The model under review builds one solid part; all positions refer to its coordinate system, in mm. A direction names the side the tool comes from. Give positions to 0.01 mm unless a question says otherwise; leave off trailing zeros. Order: outer loops, then holes, each group sorted by start corner. A loop starts at its lowest first (then second) coordinate and runs counter-clockwise, first axis right, second up. Notation, with made-up numbers: (-36, 3.25) - (-13, 3.25) arc R17 cw to (-13, 26.25) - close; hole circle Ø5 at (16, 65). An arc over 180 degrees is marked (long way). Use CSV: the item, a comma, the result in double quotes. Start each with the question number.
```python
from build123d import *


with BuildPart() as part:
    # Sketch1 → Revolve1 (revolve)
    with BuildSketch(Plane.XY, mode=Mode.PRIVATE) as revolve1_sk:
        with BuildLine():
            Line((0, 0), (2.9, 0))
            Line((2.9, 0), (2.9, 7.9))
            Line((2.9, 7.9), (8.732864907, 7.9))
            Line((8.732864907, 7.9), (8.732864907, 8.57))
            Line((8.732864907, 8.57), (2.9, 8.57))
            Line((2.9, 8.57), (2.9, 29.97))
            Line((2.9, 29.97), (1.9, 29.97))
            Line((1.9, 29.97), (2.5, 35.07))
            Line((2.5, 35.07), (1.5, 35.07))
            Line((1.5, 35.07), (1.5, 66.323834281))
            ThreePointArc((1.5, 66.323834281), (1.107157772, 68.124815809), (0, 69.598607228))
            Line((0, 69.598607228), (0, 0))
        make_face()
    revolve(revolve1_sk.sketch.rotate(Axis((0, 69.598607228, 0), (0, -1, 0)), 90), axis=Axis((0, 69.598607228, 0), (0, -1, 0)))


solid = part.part
```
1. Consider section D-D (y = 65). Give the boundary of the cut face in (x, z), and give its area (3 significant figures).
2. Mouldability with a two-part tool opening along Y and no side actions: class faces 4 (the face through (-0.1, 19.4, -2.9)), 5 (the face through (2.15, 32.56, -0.48)), 6 (the face through (0, 35.07, 2)) as pulls with the +Y half, pulls with the -Y half, needs draft (parallel to the pull), parting line crosses it, or undercut.
3. Consider section B-B (z = 6.75). Give the boundary of the cut face in (x, y).
4. Consider section C-C (x = -6.5). Give the boundary of the cut face in (y, z), and give its area (3 significant figures).
5. Clearance check with flat-ended pins moving along their axes: pin 1 (5 mm diameter, centred on x = 5.5, z = -5, fed in from +Y); pin 2 (4 mm diameter, centred on y = 13, z = -6.5, fed in from +X); pin 3 (5 mm diameter, centred on x = 2.5, z = 1, fed in from +Y); pin 4 (1 mm diameter, centred on x = 6.5, z = 4.5, fed in from -Y). State where each tip first meets the part, or that it passes through.
6. To check wall thickness, follow L1, parallel to Y at x = 3, z = -7; L2, parallel to Y at x = 0.5, z = -2.75; L3, parallel to Z at x = 2, y = 20. State the ranges of each line that lie inside material, in increasing order. Write a range as [from, to].
7. Tool access review of faces 1 (the face through (-0.45, 50.92, 1.43)), 2 (the face through (0, 7.9, -4)), 3 (the face through (2, 29.97, 1)): name each direction out of +Z, -Z, +X, -X, +Y, -Y from which nothing blocks a thin tool from reaching the whole face with its end or side.
8. Consider section A-A (y = 24.5). Give the boundary of the cut face in (x, z).
Answers follow:
1,outline,"circle Ø3 at (0, 0)"
1,area,"7.07 mm^2"
2,face 4,"needs draft"
2,face 5,"undercut"
2,face 6,"pulls with the +Y half"
3,outline,"(-5.54, 7.9) - (5.54, 7.9) - (5.54, 8.57) - (-5.54, 8.57) - close"
4,outline,"(7.9, -5.83) - (8.57, -5.83) - (8.57, 5.83) - (7.9, 5.83) - close"
4,area,"7.81 mm^2"
5,pin 1,"stops at y = 8.57"
5,pin 2,"passes through"
5,pin 3,"stops at y = 69.42"
5,pin 4,"stops at y = 7.9"
6,L1,"y = [7.9, 8.57]"
6,L2,"y = [0, 29.97]"
6,L3,"z = [-2.1, 2.1]"
7,face 1,"+Y"
7,face 2,"-Y"
7,face 3,"none"
8,outline,"circle Ø5.8 at (0, 0)"
